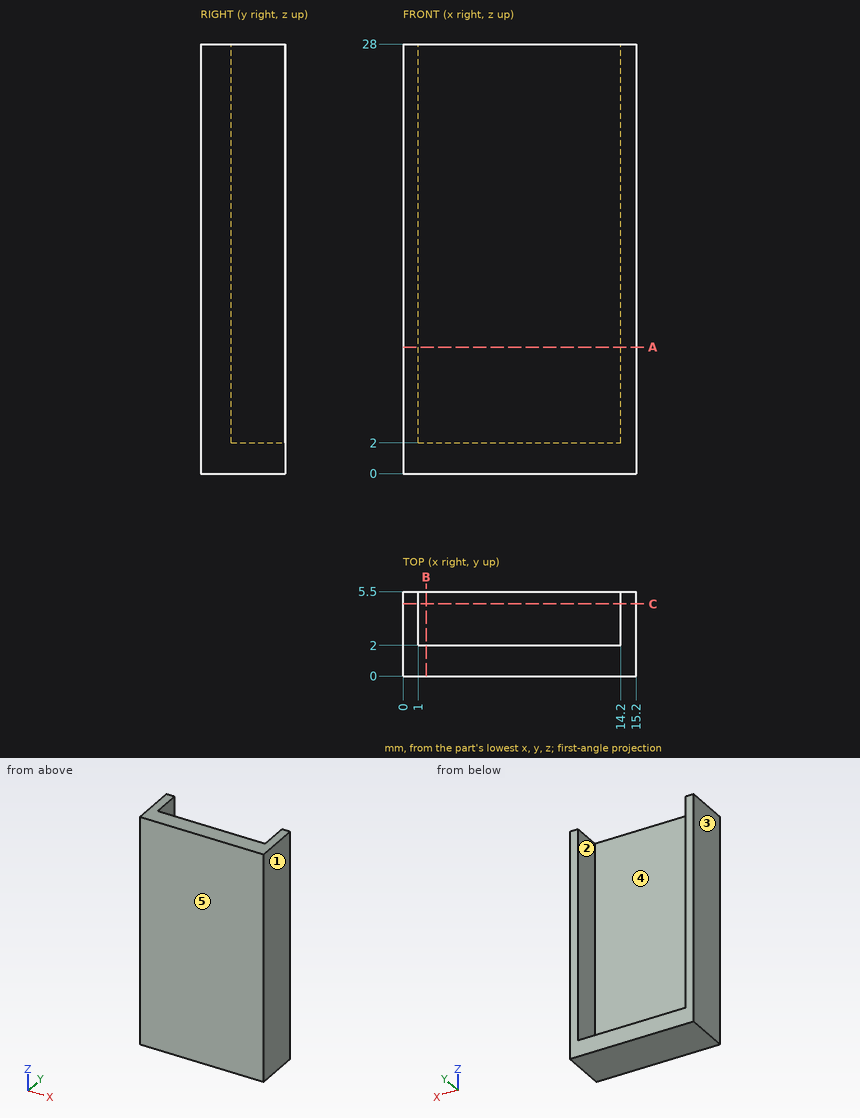
Geometry: see drawing. Coordinates: mm, zero at the bounding-box minimum. A direction names the side the tool comes from. Round coordinates to 2 decimals unless told otherwise and drop trailing zeros. Loops run counter-clockwise (first coordinate to the right, second up) from the corner with the lowest first, then second, coordinate; pieces in that order, holes last. Notation, with made-up numbers: (-27, 12) -> (1, 12) arc R34 ccw to (1, 43) -> close; hole circle Ø3 at (-12, 34). An arc over 180 degrees is marked (long way). Use one line per item in the form item = value. Start each with the question number.
Item 1: Mould query, pull axis X, two halves, no side actions, for the marked faces 3, 4 and 5. Classes: pulls with the +X half, pulls with the -X half, needs draft (parallel to the pull), parting line crosses it, or undercut.
Item 2: Contact query for flat-ended pins moving along their axis: pin 1 Ø1 at (x, y) = (6.5, 5) entering from +Z; pin 2 Ø6.5 at (x, z) = (9.5, 11.5) entering from +Y. Output: stop coordinate, or through.
Item 3: Section query B-B on x = 1.5. Return the cut outline in (y, z), then the cut area to 3 significant figures.
Item 4: Section query A-A on z = 8.25. Return the cut outline in (x, y).
Item 5: Set-up query: the marked faces 1 and 2. Return all of +Z, -Z, +X, -X, +Y, -Y with unobstructed straight access to the full face (end or side cutting, diameter ignored); none if empty.
Item 6: Section query C-C on y = 4.7. Return the cut outline in (x, z), then the cut area to 3 significant figures.
Item 7: Material intervals for L1, parallel to X at y = 5, z = 3.75; L2, parallel to Y at x = 13.75, z = 18, sorted ascending. Write a range as from..to.
Ans:
q1.face_3 = pulls with the -X half
q1.face_4 = undercut
q1.face_5 = needs draft
q2.pin_1 = 2
q2.pin_2 = 2
q3.outline = (0, 0) -> (5.5, 0) -> (5.5, 2) -> (2, 2) -> (2, 28) -> (0, 28) -> close
q3.area = 63.0 mm^2
q4.outline = (0, 0) -> (15.2, 0) -> (15.2, 5.5) -> (14.2, 5.5) -> (14.2, 2) -> (1, 2) -> (1, 5.5) -> (0, 5.5) -> close
q5.face_1 = +Z, -Z, +X, +Y, -Y
q5.face_2 = +Z, +Y
q6.outline = (0, 0) -> (15.2, 0) -> (15.2, 28) -> (14.2, 28) -> (14.2, 2) -> (1, 2) -> (1, 28) -> (0, 28) -> close
q6.area = 82.4 mm^2
q7.L1 = 0..1, 14.2..15.2
q7.L2 = 0..2
